Verification items for the finished model (mm, model axes). A direction names the side the tool comes from. Coordinates: 2 decimals unless noted, no trailing zeros. Loops run counter-clockwise (first coordinate to the right, second up) from the corner with the lowest first, then second, coordinate; pieces in that order, holes last.
Q1. Material ranges on probe 1 along Y at (x, z) = (25.5, 1.05); probe 2 along X at (y, z) = (-7, 5.5); probe 3 along Y at (x, z) = (18, 5), recorded low to high.
Q2. Sectioned sample at A-A (x = 25.5). Enter the section's corners in (y, z).
Q3. Go/stop test with flat-tipped pins: P1, Ø4, axis at x = 10.5, y = -0.5, coming from the +Z side; P2, Ø2, axis at x = -6.5, z = 4, coming from the +Y side; P3, Ø6, axis at y = -5.5, z = 8.5, coming from the +X side. Record where each tip stops, or that it passes through.
Q4. Mould release check, pull along Y, two halves, no side actions. Record for faces 1 (the face through (25.292, 17.586, 0.789)), 2 (the face through (-16, 0, 23.4)), 3 (the face through (0, 19, 1)): +Y half, -Y half, draft (parallel to the pull), parting line (faces both ways), or undercut.
Q5. Sectioned sample at C-C (x = -10.5). Enter the section's corners in (y, z).
Q6. Sectioned sample at B-B (z = 9). Enter the section's corners in (x, y), then the cut area to 3 significant figures.
Q7. Access from +Z, -Z, +X, -X, +Y, -Y to the whole of each face (thin tool, end or side, straight path). Record for faces 4 (the face through (-23.199, 0, 12)), 5 (the face through (-16, 8.331, 12)), 6 (the face through (-8.276, -7, 9)), 7 (the face through (21.374, 7, 9)).
Q8. Sectioned sample at D-D (y = 5). Enter the section's corners in (x, z).
```python
from build123d import *

# Parameters (mm, degrees)
SKETCH1_W           = 57
SKETCH1_H           = 38
SKETCH1_R           = 1.6
BOSS_EXTRUDE1_DEPTH = 1.6
SKETCH2_W           = 13.757535131
SKETCH2_H           = 16.66221661
SKETCH2_W_2         = 29.650373418
SKETCH2_H_2         = 11.582071503
BOSS_EXTRUDE2_DEPTH = 21.8
SKETCH3_W           = 29.650373418
SKETCH3_H           = 6.677072175
CUT_EXTRUDE1_DEPTH  = 49.551387626


with BuildPart() as part:
    # Sketch1 → Boss-Extrude1 (new body)
    with BuildSketch(Plane.XY):
        Rectangle(SKETCH1_W, SKETCH1_H)
        with Locations((-25.5, 16)):
            Circle(SKETCH1_R, mode=Mode.SUBTRACT)
        with Locations((-25.5, -16)):
            Circle(SKETCH1_R, mode=Mode.SUBTRACT)
        with Locations((25.5, -16)):
            Circle(SKETCH1_R, mode=Mode.SUBTRACT)
        with Locations((25.5, 16)):
            Circle(SKETCH1_R, mode=Mode.SUBTRACT)
    extrude(amount=BOSS_EXTRUDE1_DEPTH)

    # Sketch2 → Boss-Extrude2 (add)
    with BuildSketch(Plane.XY.offset(1.6)):
        with Locations((-16.320596847, 0)):
            Rectangle(SKETCH2_W, SKETCH2_H)
        with Locations((6.548865085, 6.791035752)):
            Rectangle(SKETCH2_W_2, SKETCH2_H_2)
        with Locations((6.548865085, -6.791035752)):
            Rectangle(SKETCH2_W_2, SKETCH2_H_2)
    extrude(amount=BOSS_EXTRUDE2_DEPTH)

    # Sketch3 → Cut-Extrude1 (cut, through all)
    with BuildSketch(Plane(origin=(0, -12.582071503, 0), x_dir=(-1, 0, 0), z_dir=(0, -1, 0))):
        with Locations((-6.548865085, -20.061463913)):
            Rectangle(SKETCH3_W, SKETCH3_H)
    extrude(amount=-CUT_EXTRUDE1_DEPTH, mode=Mode.SUBTRACT)


solid = part.part
```
Geometry check:
1. probe 1: y = -19 to -17.6, -14.4 to 14.4, 17.6 to 19
1. probe 2: x = -23.2 to -9.44, -8.28 to 21.37
1. probe 3: y = -12.58 to -1, 1 to 12.58
2. outline: (-19, 0) - (-17.6, 0) - (-17.6, 1.6) - (-19, 1.6) - close; (-14.4, 0) - (14.4, 0) - (14.4, 1.6) - (-14.4, 1.6) - close; (17.6, 0) - (19, 0) - (19, 1.6) - (17.6, 1.6) - close
3. P1: stops at z = 16.72
3. P2: stops at y = 12.58
3. P3: stops at x = 21.37
4. face 1: undercut
4. face 2: draft
4. face 3: +Y half
5. outline: (-19, 0) - (19, 0) - (19, 1.6) - (8.33, 1.6) - (8.33, 23.4) - (-8.33, 23.4) - (-8.33, 1.6) - (-19, 1.6) - close
6. outline: (-23.2, -8.33) - (-9.44, -8.33) - (-9.44, 8.33) - (-23.2, 8.33) - close; (-8.28, -12.58) - (21.37, -12.58) - (21.37, -1) - (-8.28, -1) - close; (-8.28, 1) - (21.37, 1) - (21.37, 12.58) - (-8.28, 12.58) - close
6. area: 916 mm2
7. face 4: +Z, -X, +Y, -Y
7. face 5: +Z, -X, +Y
7. face 6: +Z, +Y, -Y
7. face 7: +Z, +X, +Y, -Y
8. outline: (-28.5, 0) - (28.5, 0) - (28.5, 1.6) - (21.37, 1.6) - (21.37, 16.72) - (-8.28, 16.72) - (-8.28, 1.6) - (-9.44, 1.6) - (-9.44, 23.4) - (-23.2, 23.4) - (-23.2, 1.6) - (-28.5, 1.6) - close
